```python
from build123d import *

# Parameters (mm, degrees)
F1_DEPTH = 4.5
F2_W     = 28.5
F2_H     = 4.5
F2_R     = 2.5
F2_W_2   = 25
F2_H_2   = 100
F2_W_3   = 50
F2_H_3   = 25
F2_W_4   = 83
F2_H_4   = 86
F3_DEPTH = 25


with BuildPart() as f1:
    # F0 (on Top) → F1 (new body)
    with BuildSketch(Plane.XY):
        with BuildLine():
            Line((104.879995, 146.808884), (-109.120005, 146.808884))
            ThreePointArc((-109.120005, 146.808884), (-119.0195, 142.708379), (-123.120005, 132.808884))
            Line((-123.120005, 132.808884), (-123.120005, -178.191116))
            ThreePointArc((-123.120005, -178.191116), (-119.0195, -188.090611), (-109.120005, -192.191116))
            Line((-109.120005, -192.191116), (104.879995, -192.191116))
            ThreePointArc((104.879995, -192.191116), (114.77949, -188.090611), (118.879995, -178.191116))
            Line((118.879995, -178.191116), (118.879995, 132.808884))
            ThreePointArc((118.879995, 132.808884), (114.77949, 142.708379), (104.879995, 146.808884))
        make_face()
        with BuildLine():
            ThreePointArc((-65.620005, 117.308884), (-61.812393, 126.501272), (-52.620005, 130.308884))
            Line((-52.620005, 130.308884), (48.379995, 130.308884))
            ThreePointArc((48.379995, 130.308884), (57.572383, 126.501272), (61.379995, 117.308884))
            ThreePointArc((61.379995, 117.308884), (57.572383, 108.116496), (48.379995, 104.308884))
            Line((48.379995, 104.308884), (-52.620005, 104.308884))
            ThreePointArc((-52.620005, 104.308884), (-61.812393, 108.116496), (-65.620005, 117.308884))
        make_face(mode=Mode.SUBTRACT)
    extrude(amount=F1_DEPTH)

    # F2 (on face) → F3 (cut)
    with BuildSketch(Plane.XY.offset(4.5)):
        with Locations((-90.370005, 47.058884)):
            Rectangle(F2_W, F2_H)
        with Locations((-116.120005, 24.308884)):
            Circle(F2_R)
        with Locations((-116.120005, 12.308884)):
            Circle(F2_R)
        with Locations((-116.120005, -57.691116)):
            Circle(F2_R)
        with Locations((-116.120005, -69.691116)):
            Circle(F2_R)
        with Locations((-90.370005, -92.441116)):
            Rectangle(F2_W, F2_H)
        with Locations((86.129995, 47.058884)):
            Rectangle(F2_W, F2_H)
        with Locations((86.129995, -92.441116)):
            Rectangle(F2_W, F2_H)
        with Locations((111.879995, 24.308884)):
            Circle(F2_R)
        with Locations((111.879995, 12.308884)):
            Circle(F2_R)
        with Locations((111.879995, -57.691116)):
            Circle(F2_R)
        with Locations((111.879995, -69.691116)):
            Circle(F2_R)
        with Locations((-84.620005, -22.691116)):
            Rectangle(F2_W_2, F2_H_2)
        with Locations((-98.120005, 101.808884)):
            Rectangle(F2_W_3, F2_H_3)
        with Locations((-98.120005, -147.191116)):
            Rectangle(F2_W_3, F2_H_3)
        with Locations((-2.120005, 103.808884)):
            Rectangle(F2_W_4, F2_H_4)
        with Locations((-2.120005, -149.191116)):
            Rectangle(F2_W_4, F2_H_4)
    extrude(amount=-F3_DEPTH, mode=Mode.SUBTRACT)


solid = f1.part
```
Build history of the part. All positions in model axes, mm. Round coordinates to 2 decimals unless told otherwise and drop trailing zeros. Write each loop counter-clockwise with the first axis right and the second up, starting at its lowest first coordinate (ties: lowest second). Pieces come first, ordered by that corner, then holes. Notation, with made-up numbers: (-14, 79.25) -> (24, 79.25) arc R31 cw to (24, 110.25) -> close; hole circle Ø4 at (74.5, 75). An arc over 180 degrees is marked (long way). Put each result on its own line as item: value.
Item 1: Slice it at C-C, the plane x = -86. Give the cut face in (y, z), plus the area to 3 significant figures.
Here are the results:
outline: (-192.19, 0) -> (-159.69, 0) -> (-159.69, 4.5) -> (-192.19, 4.5) -> close; (-134.69, 0) -> (-94.69, 0) -> (-94.69, 4.5) -> (-134.69, 4.5) -> close; (-90.19, 0) -> (-72.69, 0) -> (-72.69, 4.5) -> (-90.19, 4.5) -> close; (27.31, 0) -> (44.81, 0) -> (44.81, 4.5) -> (27.31, 4.5) -> close; (49.31, 0) -> (89.31, 0) -> (89.31, 4.5) -> (49.31, 4.5) -> close; (114.31, 0) -> (146.81, 0) -> (146.81, 4.5) -> (114.31, 4.5) -> close
area: 810 mm^2
Item 2: Flat gauge pins, fed straight in: P1, Ø2, axis at x = 24.5, z = 3.5, coming from the -Y side; P2, Ø12, axis at x = 24, y = -77, coming from the -Z side; P3, Ø2, axis at y = 142.5, z = 1, coming from the -X side. Where does each tip first touch, or does it go through?
Here are the results:
P1: stops at y = -106.19
P2: stops at z = 0
P3: stops at x = -120.1
Item 3: Slice it at A-A, the plane x = 94. Give the cut face in (y, z), plus the area to 4 significant figures.
Here are the results:
outline: (-192.19, 0) -> (-94.69, 0) -> (-94.69, 4.5) -> (-192.19, 4.5) -> close; (-90.19, 0) -> (44.81, 0) -> (44.81, 4.5) -> (-90.19, 4.5) -> close; (49.31, 0) -> (146.81, 0) -> (146.81, 4.5) -> (49.31, 4.5) -> close
area: 1,485 mm^2
Item 4: Wall check: probe 1 along Y at (x, z) = (-105.5, 2.15); probe 2 along Y at (x, z) = (-91, 2.95); probe 3 along X at (y, z) = (-143, 2.2). Give the ranges that are in metal, low to high. Write a range as from..to.
Here are the results:
probe 1: y = -192.19..-159.69, -134.69..89.31, 114.31..146.81
probe 2: y = -192.19..-159.69, -134.69..-94.69, -90.19..-72.69, 27.31..44.81, 49.31..89.31, 114.31..146.81
probe 3: x = -73.12..-43.62, 39.38..118.88
Item 5: Slice it at B-B, the plane y = -0.5. Give the cut face in (x, z), plus the area to 4 significant figures.
Here are the results:
outline: (-123.12, 0) -> (-97.12, 0) -> (-97.12, 4.5) -> (-123.12, 4.5) -> close; (-72.12, 0) -> (118.88, 0) -> (118.88, 4.5) -> (-72.12, 4.5) -> close
area: 976.5 mm^2
Item 6: Slice it at D-D, the plane y = -116. Give the cut face in (x, z).
Here are the results:
outline: (-123.12, 0) -> (-43.62, 0) -> (-43.62, 4.5) -> (-123.12, 4.5) -> close; (39.38, 0) -> (118.88, 0) -> (118.88, 4.5) -> (39.38, 4.5) -> close
